Source: CAD feature listing. Evaluate the final solid. Frame: model axes, mm. Face numbers are marked on the shaded views. Round coordinates to 2 decimals unless told otherwise and drop trailing zeros. Order: outer loops, then holes, each group sorted by start corner. A loop starts at its lowest first (then second) coordinate and runs counter-clockwise, first axis right, second up.
```python
from build123d import *

# Parameters (mm, degrees)
ESQUISSE1_W                                 = 145.148196
ESQUISSE1_H                                 = 60
BOSS_EXTRU_1_DEPTH                          = 1.5
BOSS_EXTRU_2_DEPTH                          = 2
FRAISAGE_POUR_VIS_T_TE_FRAIS_E_M31_AT_COUNT = 2
FRAISAGE_POUR_VIS_T_TE_FRAIS_E_M31_AT_PITCH = 52
FRAISAGE_POUR_VIS_T_TE_FRAIS_E_M31_2_COUNT  = 2
FRAISAGE_POUR_VIS_T_TE_FRAIS_E_M31_2_PITCH  = 135.572178
FRAISAGE_POUR_VIS_T_TE_FRAIS_E_M31_3_COUNT  = 2
FRAISAGE_POUR_VIS_T_TE_FRAIS_E_M31_3_PITCH  = 145.20267025
ENL_V_MAT_EXTRU_1_DEPTH                     = 79.608203774
ENL_V_MAT_EXTRU_1_DEPTH_BACK                = 79.608203774
ESQUISSE6_W                                 = 24
ESQUISSE6_H                                 = 6
CONG_1_R                                    = 3
ESQUISSE7_W                                 = 45
ESQUISSE7_H                                 = 40
ENL_V_MAT_EXTRU_2_DEPTH                     = 2


with BuildPart() as part:
    # Esquisse1 → Boss.-Extru.1 (new body)
    with BuildSketch(Plane.XY):
        Rectangle(ESQUISSE1_W, ESQUISSE1_H)
    extrude(amount=BOSS_EXTRU_1_DEPTH)

    # Esquisse2 → Boss.-Extru.2 (add)
    with BuildSketch(Plane(origin=(0, 0, 0), x_dir=(-1, 0, 0), z_dir=(0, 0, -1))):
        with BuildLine():
            Line((-71.374098, -16.8), (-71.374098, 16.8))
            ThreePointArc((-71.374098, 16.8), (-64.303030188, 19.728932188), (-61.374098, 26.8))
            Line((-61.374098, 26.8), (61.374098, 26.8))
            ThreePointArc((61.374098, 26.8), (64.303030188, 19.728932188), (71.374098, 16.8))
            Line((71.374098, 16.8), (71.374098, -16.8))
            ThreePointArc((71.374098, -16.8), (64.303030188, -19.728932188), (61.374098, -26.8))
            Line((61.374098, -26.8), (-61.374098, -26.8))
            ThreePointArc((-61.374098, -26.8), (-64.303030188, -19.728932188), (-71.374098, -16.8))
        make_face()
    extrude(amount=BOSS_EXTRU_2_DEPTH)

    # Esquisse5 → Fraisage pour vis à tête fraisée M31 (revolve, cut)
    with BuildSketch(Plane(origin=(-68.574098, 26, 1.5), x_dir=(0, -1, 0), z_dir=(1, 0, 0))):
        Polygon((0, 0), (0, 1.5), (1.7, 1.5), (1.7, 1.45), (3.15, 0), align=None)
    fraisage_pour_vis_t_te_frais_e_m31 = revolve(axis=Axis((-68.574098, 26, 7.85), (0, 0, -1)), mode=Mode.SUBTRACT)

    # Fraisage pour vis à tête fraisée M31 at: Fraisage pour vis à tête fraisée M31 ×2
    with Locations(*[(0, -i * FRAISAGE_POUR_VIS_T_TE_FRAIS_E_M31_AT_PITCH, 0) for i in range(1, FRAISAGE_POUR_VIS_T_TE_FRAIS_E_M31_AT_COUNT)]):
        add(fraisage_pour_vis_t_te_frais_e_m31, mode=Mode.SUBTRACT)

    # Fraisage pour vis _ t_te frais_e M31 2: Fraisage pour vis à tête fraisée M31 ×2
    with Locations(*[(i * FRAISAGE_POUR_VIS_T_TE_FRAIS_E_M31_2_PITCH, 0, 0) for i in range(1, FRAISAGE_POUR_VIS_T_TE_FRAIS_E_M31_2_COUNT)]):
        add(fraisage_pour_vis_t_te_frais_e_m31, mode=Mode.SUBTRACT)

    # Fraisage pour vis _ t_te frais_e M31 3: Fraisage pour vis à tête fraisée M31 ×2
    with Locations(*[Vector(0.9336755155176905, -0.35812013588009123, 0) * (i * FRAISAGE_POUR_VIS_T_TE_FRAIS_E_M31_3_PITCH) for i in range(1, FRAISAGE_POUR_VIS_T_TE_FRAIS_E_M31_3_COUNT)]):
        add(fraisage_pour_vis_t_te_frais_e_m31, mode=Mode.SUBTRACT)

    # Esquisse6 → Enlèv. mat.-Extru.1 (cut, two sides: drawn at the far end of the back side and taken through both)
    with BuildSketch(Plane.XY.offset(1.5).offset(-ENL_V_MAT_EXTRU_1_DEPTH_BACK)):
        with Locations((-40.574098, 27)):
            Rectangle(ESQUISSE6_W, ESQUISSE6_H)
    extrude(amount=ENL_V_MAT_EXTRU_1_DEPTH + ENL_V_MAT_EXTRU_1_DEPTH_BACK, mode=Mode.SUBTRACT)

    # Congé1
    cong_1_edges = [part.edges().sort_by_distance(p)[0] for p in [
        (-28.574098, 30, 0.75),
        (-28.574098, 24, -0.25),
        (-52.574098, 30, 0.75),
        (-52.574098, 24, -0.25),
    ]]
    fillet(cong_1_edges, radius=CONG_1_R - 0.0001)  # a hair under: the kernel refuses the full size

    # Esquisse7 → Enlèv. mat.-Extru.2 (cut)
    with BuildSketch(Plane(origin=(0, 0, -2), x_dir=(-1, 0, 0), z_dir=(0, 0, -1))):
        with Locations((-13.455902, 6.8)):
            Rectangle(ESQUISSE7_W, ESQUISSE7_H)
    extrude(amount=-ENL_V_MAT_EXTRU_2_DEPTH, mode=Mode.SUBTRACT)


solid = part.part
```
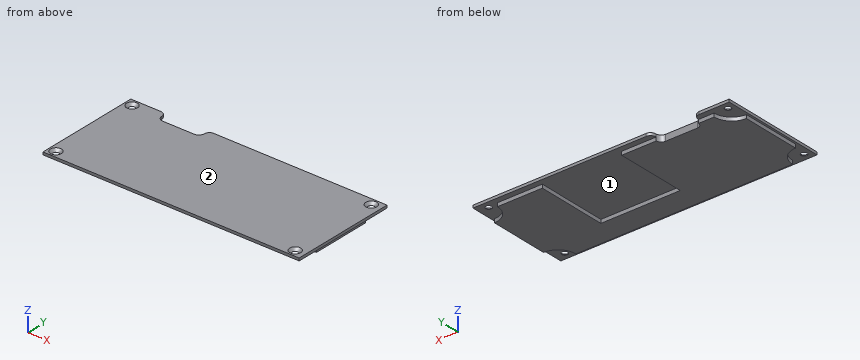
1. Line query: line 1 along X through (y, z) = (-26, 0.05); line 2 along X through (y, z) = (9, -0.3); line 3 along Y through (x, z) = (-57, -0.3). Output: solid intervals per line, ascending.
2. First-contact query: pin 1 (2.5 mm diameter, centred on x = -68.57, y = 26, fed in from +Z); pin 2 (1 mm diameter, centred on x = -45, z = 0.5, fed in from +Y); pin 3 (18 mm diameter, centred on x = 0.5, y = -4.5, fed in from -Z); pin 4 (4.5 mm diameter, centred on x = -68.57, y = -26, fed in from -Z). Flat tips, straight axial feed; report the tip coordinate or a pass-through.
3. Pull-direction query (X, two-part tool) for the marked faces 1 and 2; classes: released by +X, released by -X, zero draft, split by the parting line, or undercut.
4. Section D-D on x = 24.5. Return loops of the section in (y, z).
5. Section A-A on x = -21. Return loops of the section in (y, z), plus the area to 3 significant figures.
6. Section C-C on z = 0.7. State how many separate pieces and enclosed holes the cut face has, plus the area to 3 significant figures.
7. Section B-B on y = -4.5. Return loops of the section in (x, z).
Result:
1. line 1: x = -72.57 to -70.27, -66.87 to 65.3, 68.7 to 72.57
1. line 2: x = -71.37 to -9.04, 35.96 to 71.37
1. line 3: y = -26.8 to 26.8
2. pin 1: passes through
2. pin 2: stops at y = 24
2. pin 3: stops at z = -2
2. pin 4: stops at z = 0
3. face 1: undercut
3. face 2: zero draft
4. outline: (-30, 0) - (-26.8, 0) - (-26.8, -2) - (-13.2, -2) - (-13.2, 0) - (30, 0) - (30, 1.5) - (-30, 1.5) - close
5. outline: (-30, 0) - (-26.8, 0) - (-26.8, -2) - (26.8, -2) - (26.8, 0) - (30, 0) - (30, 1.5) - (-30, 1.5) - close
5. area: 197 mm2
6. separate pieces: 1
6. enclosed holes: 4
6. area: 8,500 mm2
7. outline: (-72.57, 0) - (-71.37, 0) - (-71.37, -2) - (-9.04, -2) - (-9.04, 0) - (35.96, 0) - (35.96, -2) - (71.37, -2) - (71.37, 0) - (72.57, 0) - (72.57, 1.5) - (-72.57, 1.5) - close
